```python
from build123d import *

# Parameters (mm, degrees)
BOSS_EXTRUDE3_DEPTH = 7.75
SKETCH4_R           = 3
BOSS_EXTRUDE4_DEPTH = 3


with BuildPart() as part:
    # Sketch3 → Boss-Extrude3 (new body)
    with BuildSketch(Plane.XY):
        Polygon((-2.5, 5), (2.5, 5), (2.5, -5), (-2.5, -5), (-23.713203436, -26.213203436), (-28.713203436, -21.213203436), (-7.5, 0), (-38.612698372, 31.112698372), (-33.612698372, 36.112698372), align=None)
    extrude(amount=BOSS_EXTRUDE3_DEPTH)

    # Sketch4 → Boss-Extrude4 (add)
    with BuildSketch(Plane(origin=(2.5, 0, 0), x_dir=(0, 0, -1), z_dir=(1, 0, 0))):
        with Locations(Location((-3.875, 0, 0), (0, 0, 90))):
            Circle(SKETCH4_R)
    extrude(amount=BOSS_EXTRUDE4_DEPTH)

    # Sketch5 → Revolve1 (revolve)
    with BuildSketch(Plane(origin=(5.5, 0, 0), x_dir=(0, 0, -1), z_dir=(1, 0, 0))):
        with BuildLine():
            Line((-3.875, 3.75), (-3.875, -3.75))
            ThreePointArc((-3.875, -3.75), (-7.625, 0), (-3.875, 3.75))
        make_face()
    revolve(axis=Axis((5.5, 4.135747614, 3.875), (0, -1, 0)))


solid = part.part
```
CAD build for the part. Positions are in the model's coordinates, mm. A direction names the side the tool comes from. Coordinates: 2 decimals unless noted, no trailing zeros. Order: outer loops, then holes, each group sorted by start corner. A loop starts at its lowest first (then second) coordinate and runs counter-clockwise, first axis right, second up. Notation, with made-up numbers: M 46,17.25 L 105,17.25 A19 cw 105,35.25 Z; hole C 3.25,-2 d9. An arc over 180 degrees is marked long. Write each question's results on one line, items separated by ' | '. Start each with the question number.
Q1. Drill centre lines: probe 1 along Y at (x, z) = (0.5, 4); probe 2 along Y at (x, z) = (-8, 1.5); probe 3 along Y at (x, z) = (-28, 6.25). Where is each one in solid material? Low to high. Write a range as from..to.
Q2. Cut at D-D (x = -31). List the corners of the cut face in (y, z).
Q3. Cut at A-A (x = -9.5). List the corners of the cut face in (y, z).
Q4. Cut at C-C (y = 15.5). List the corners of the cut face in (x, z).
Q5. Cut at B-B (z = 1.75). List the corners of the cut face in (x, y).
Q6. Pull direction X, two halves, no side cores. Call faces 4 (the flat face through (2.5, 3.4, 3.8)), 5 (the flat face through (-36.148, 33.578, 3.821)), 6 (the flat face through (-13, 7, 0)): +X half, -X half, draft (parallel to the pull), parting line (faces both ways), or undercut.
Q7. Which spindle directions (+Z, -Z, +X, -X, +Y, -Y) get a long thin tool onto all of the face, cutting with end or side? Do faces 1 (the cylindrical face through (2.87, 2.771, 2.726)), 2 (the flat face through (-22.8, 15.3, 3.8)), 3 (the flat face through (0, 5, 4)). Say none if no direction does.
Q8. Flat gauge pins, fed straight in: P1, Ø4, axis at x = 1, z = 4, coming from the +Y side; P2, Ø4, axis at x = -10.5, z = 6.5, coming from the +Y side; P3, Ø1, axis at x = 1.5, z = 2.5, coming from the -Y side. Where does each tip first touch, or does it go through?
Found:
1) probe 1: -5..5 | probe 2: -10.5..-0.5, 0.5..10.5 | probe 3: -21.93..-20.5, 20.5..30.5
2) outline: M 23.5,0 L 33.5,0 L 33.5,7.75 L 23.5,7.75 Z
3) outline: M -12,0 L -2,0 L -2,7.75 L -12,7.75 Z; M 2,0 L 12,0 L 12,7.75 L 2,7.75 Z
4) outline: M -23,0 L -13,0 L -13,7.75 L -23,7.75 Z
5) outline: M -38.61,31.11 L -7.5,0 L -28.71,-21.21 L -23.71,-26.21 L -2.5,-5 L 2.5,-5 L 2.5,-2.12 L 3.25,-2.12 A3.09 ccw long 3.25,2.12 L 2.5,2.12 L 2.5,5 L -2.5,5 L -33.61,36.11 Z
6) face 4: undercut | face 5: -X half | face 6: draft
7) face 1: none | face 2: +Z, -Z, -X | face 3: +Z, -Z, +X, +Y
8) P1: y = 5 | P2: y = 15 | P3: y = -5
